from build123d import *

# Parameters (mm, degrees)
F0_R      = 9.525
F0_R_2    = 4.826
F1_DEPTH  = 12.954
F2_R      = 4.1275
F3_DEPTH  = 6.35
F5_R      = 1.5875
F6_DEPTH  = 31.75
F7_DEPTH  = 25.4
F8_R      = 6.35
F9_DEPTH  = 1.27
F5_R_2    = 4.445
F10_DEPTH = 17.78
F11_R     = 2.54


with BuildPart() as f1:
    # F0 (on Top) → F1 (new body)
    with BuildSketch(Plane.XY):
        Circle(F0_R)
        Circle(F0_R_2, mode=Mode.SUBTRACT)
    extrude(amount=F1_DEPTH)

    # F2 (on face) → F3 (join)
    with BuildSketch(Plane.XY.offset(12.954)):
        with BuildLine():
            ThreePointArc((-0.3406139649, -9.5189078747), (6.6136705763, -6.8545595415), (9.525, 0))
            ThreePointArc((9.525, 0), (6.6137479521, 6.8544848841), (-0.3403990606, 9.5189155622))
            ThreePointArc((-0.3403990606, 9.5189155622), (-9.5249999994, 0.0001075209), (-0.3406139649, -9.5189078747))
        make_face()
        with BuildLine():
            ThreePointArc((-0.3406139649, -9.5189078747), (-9.5249999994, 0.0001075209), (-0.3403990606, 9.5189155622))
            Line((-0.3403990606, 9.5189155622), (-88.965388203, 6.3496633283))
            ThreePointArc((-88.965388203, 6.3496633283), (-84.4330499829, 4.5131870717), (-82.55, 0))
            ThreePointArc((-82.55, 0), (-84.4098719395, -4.4901280605), (-88.9, -6.35))
            Line((-88.9, -6.35), (-0.3406139649, -9.5189078747))
        make_face()
        with Locations((-76.581, 0)):
            Circle(F2_R, mode=Mode.SUBTRACT)
        with Locations((-64.262, 0)):
            Circle(F2_R, mode=Mode.SUBTRACT)
        with Locations((-51.943, 0)):
            Circle(F2_R, mode=Mode.SUBTRACT)
        with Locations((-39.624, 0)):
            Circle(F2_R, mode=Mode.SUBTRACT)
        with Locations((-27.305, 0)):
            Circle(F2_R, mode=Mode.SUBTRACT)
        with Locations((-14.986, 0)):
            Circle(F2_R, mode=Mode.SUBTRACT)
        with BuildLine():
            ThreePointArc((-82.55, 0), (-84.4330499829, 4.5131870717), (-88.965388203, 6.3496633283))
            ThreePointArc((-88.965388203, 6.3496633283), (-95.2499158315, -0.0326945349), (-88.9, -6.35))
            ThreePointArc((-88.9, -6.35), (-84.4098719395, -4.4901280605), (-82.55, 0))
        make_face()
        with Locations((-88.9, 0)):
            Circle(F2_R, mode=Mode.SUBTRACT)
    extrude(amount=-F3_DEPTH)

    # F5 (on offset) → F6 (cut)
    with BuildSketch(Plane.YZ.offset(25.4)):
        with Locations((0, 6.096)):
            Circle(F5_R)
    extrude(amount=-F6_DEPTH, mode=Mode.SUBTRACT)

    # F0 (on Top) → F7 (cut)
    with BuildSketch(Plane.XY):
        Circle(F0_R_2)
    extrude(amount=F7_DEPTH, mode=Mode.SUBTRACT)

    # F8 (on face) → F9 (cut)
    with BuildSketch(Plane(origin=(0, 0, 6.604), x_dir=(1, 0, 0), z_dir=(0, 0, -1))):
        with Locations((-88.9, 0)):
            Circle(F8_R)
    extrude(amount=-F9_DEPTH, mode=Mode.SUBTRACT)

    # F5 (on offset) → F10 (cut)
    with BuildSketch(Plane.YZ.offset(25.4)):
        with Locations((0, 6.096)):
            Circle(F5_R_2)
        with Locations((0, 6.096)):
            Circle(F5_R, mode=Mode.SUBTRACT)
    extrude(amount=-F10_DEPTH, mode=Mode.SUBTRACT)

    # F11
    f11_edges = [f1.edges().sort_by_distance(p)[0] for p in [
        (-88.9, -6.35, 10.414),
        (-88.9, -6.35, 7.239),
        (-88.965388, 6.349663, 10.414),
        (-88.965388, 6.349663, 7.239),
    ]]
    fillet(f11_edges, radius=F11_R)


solid = f1.part
Design review of the part built by this model. Coordinates are the model's own, in mm. A direction names the side the tool comes from. Coordinates: 2 decimals unless noted, no trailing zeros. Loops run counter-clockwise (first coordinate to the right, second up) from the corner with the lowest first, then second, coordinate; pieces in that order, holes last. Notation, with made-up numbers: (-40, -29) -> (-4, -29) arc R28 cw to (-4, 2) -> close; hole circle Ø9 at (3.5, 47.5). An arc over 180 degrees is marked (long way). Use a Markdown table: item, result. Add a question column.
Item 1: Clearance check with flat-ended pins moving along their axes: P1, Ø1.5, axis at x = -68, y = -5.5, coming from the -Z side; P2, Ø8.5, axis at x = 0, y = 0, coming from the -Z side; P3, Ø2.5, axis at y = 1.5, z = 4, coming from the +X side. State where each tip first meets the part, or that it passes through.
Item 2: We need section D-D, the plane x = -53.5. Write out the cut boundary in (y, z).
Item 3: The part is to be moulded in two halves that separate along X. For faces 1 (the flat face through (-6.35, 0, 6)), 2 (the cylindrical face through (4.458, -1.848, 6.386)), 3 (the cylindrical face through (-23.5, -1.6, 9.8)), 4 (the cylindrical face through (-83.183, 5.404, 7.23)), say which applies: +X half, -X half, draft (parallel to the pull), parting line (faces both ways), or undercut.
Item 4: Machinability: for faces 5 (the cylindrical face through (-83.182, -5.402, 7.23)), 6 (the cylindrical face through (4.4, -8.45, 4.95)), 7 (the cylindrical face through (8.374, -0.964, 1.757)), which of the approach directions +Z, -Z, +X, -X, +Y, -Y give a long, thin tool a straight path to every point of the face, cutting with its end or side? Answer none if there is none.
Item 5: We need section B-B, the plane y = 0. Count the separate pieces of the cut face and the enclosed holes in it, and give its area (3 significant figures).
Item 6: We need section A-A, the plane x = -38. Write out the cut boundary in (y, z).
Item 7: Wall thickness on L1, parallel to Z at x = 6.1, y = 0; L2, parallel to Z at x = -79.5, y = 3.75; L3, parallel to Y at x = -50, z = 10.5: over which ranges is each line inside the solid? List them lowest first. Write a range as from..to.
Numbers:
| question | item | result |
|---|---|---|
| 1 | P1 | stops at z = 6.6 |
| 1 | P2 | passes through |
| 1 | P3 | stops at x = 7.62 |
| 2 | outline | (-7.62, 6.6) -> (-3.82, 6.6) -> (-3.82, 12.95) -> (-7.62, 12.95) -> close; (3.82, 6.6) -> (7.62, 6.6) -> (7.62, 12.95) -> (3.82, 12.95) -> close |
| 3 | face 1 | +X half |
| 3 | face 2 | undercut |
| 3 | face 3 | undercut |
| 3 | face 4 | -X half |
| 4 | face 5 | -Z, -X |
| 4 | face 6 | -Z |
| 4 | face 7 | +X |
| 5 | separate pieces | 10 |
| 5 | enclosed holes | 0 |
| 5 | area | 263 mm^2 |
| 6 | outline | (-8.17, 6.6) -> (-3.79, 6.6) -> (-3.79, 12.95) -> (-8.17, 12.95) -> close; (3.79, 6.6) -> (8.17, 6.6) -> (8.17, 12.95) -> (3.79, 12.95) -> close |
| 7 | L1 | z = 0..4.51, 7.68..12.95 |
| 7 | L2 | z = 6.6..12.95 |
| 7 | L3 | y = -7.74..-3.64, 3.64..7.74 |
